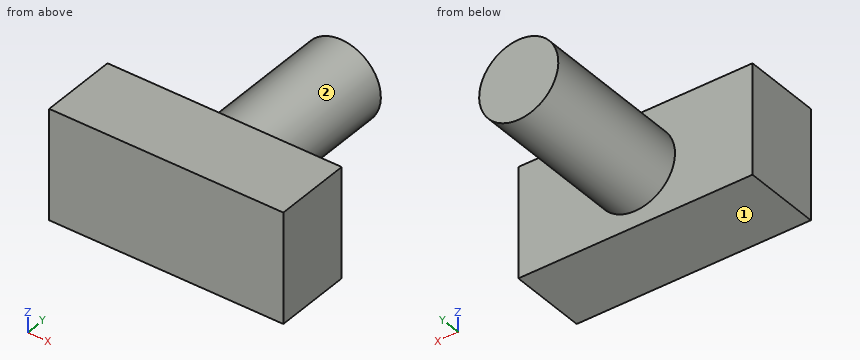
```python
from build123d import *

# Parameters (mm, degrees)
SKETCH_2_W      = 302.180498412
SKETCH_2_H      = 142.083514116
EXTRUDE_1_DEPTH = 100
SKETCH_2_3_R    = 51.07818505
EXTRUDE_2_DEPTH = 300


with BuildPart() as part:
    # Sketch 2 → Extrude 1 (new body)
    with BuildSketch(Plane(origin=(0, 0, 0), x_dir=(1, 0, 0), z_dir=(0, 1, 0))):
        Rectangle(SKETCH_2_W, SKETCH_2_H)
    extrude(amount=EXTRUDE_1_DEPTH)

    # Sketch 2_3 → Extrude 2 (add)
    with BuildSketch(Plane(origin=(0, 0, 0), x_dir=(1, 0, 0), z_dir=(0, 1, 0))):
        with Locations(Location((0, 0, 0), (0, 0, 90))):
            Circle(SKETCH_2_3_R)
    extrude(amount=EXTRUDE_2_DEPTH)


solid = part.part
```
CAD build for the part. Positions are in the model's coordinates, mm. Face numbers are marked on the shaded views. A direction names the side the tool comes from. Round coordinates to 2 decimals unless told otherwise and drop trailing zeros. Order: outer loops, then holes, each group sorted by start corner. A loop starts at its lowest first (then second) coordinate and runs counter-clockwise, first axis right, second up. Notation, with made-up numbers: (6.5, 61) - (38.5, 61) arc R26 ccw to (38.5, 92) - close; hole circle Ø6 at (65.25, -17.75). An arc over 180 degrees is marked (long way). Answer as CSV lines item,"result". Start each with the question number.
1. Saw through at B-B, the plane z = 18. Write the cut outline in (x, y), and give its area (3 significant figures).
2. Saw through at A-A, the plane x = 0. Write the cut outline in (y, z), and give its area (3 significant figures).
3. Pin check, flat tips, straight feed: pin 1 (12 mm diameter, centred on x = 9.5, y = 208, fed in from +Z); pin 2 (5 mm diameter, centred on x = 85, z = 2.5, fed in from +Y); pin 3 (6 mm diameter, centred on y = 226.5, z = 28, fed in from -X). Stop position of each tip, or through.
4. Tool access for the marked faces 1 and 2: list every direction of +Z, -Z, +X, -X, +Y, -Y with a clear straight run to the whole face (end or side of a thin tool).
5. Drill centre lines: L1, parallel to Y at x = 82, z = 53; L2, parallel to X at y = 169, z = 32; L3, parallel to X at y = 192.5, z = 13.5. Where is each one in solid material? Low to high. Write a range as [from, to].
6. Saw through at C-C, the plane y = 273. Write the cut outline in (x, z).
7. Saw through at D-D, the plane x = -118. Write the cut outline in (y, z), and give its area (3 significant figures).
Model answer:
1,outline,"(-151.09, 0) - (151.09, 0) - (151.09, 100) - (47.8, 100) - (47.8, 300) - (-47.8, 300) - (-47.8, 100) - (-151.09, 100) - close"
1,area,"49,300 mm²"
2,outline,"(0, -71.04) - (100, -71.04) - (100, -51.08) - (300, -51.08) - (300, 51.08) - (100, 51.08) - (100, 71.04) - (0, 71.04) - close"
2,area,"34,600 mm²"
3,pin 1,"stops at z = 50.96"
3,pin 2,"stops at y = 100"
3,pin 3,"stops at x = -44.54"
4,face 1,"-Z, +X, -X, +Y, -Y"
4,face 2,"+Y"
5,L1,"y = [0, 100]"
5,L2,"x = [-39.81, 39.81]"
5,L3,"x = [-49.26, 49.26]"
6,outline,"circle Ø102.16 at (0, 0)"
7,outline,"(0, -71.04) - (100, -71.04) - (100, 71.04) - (0, 71.04) - close"
7,area,"14,200 mm²"
